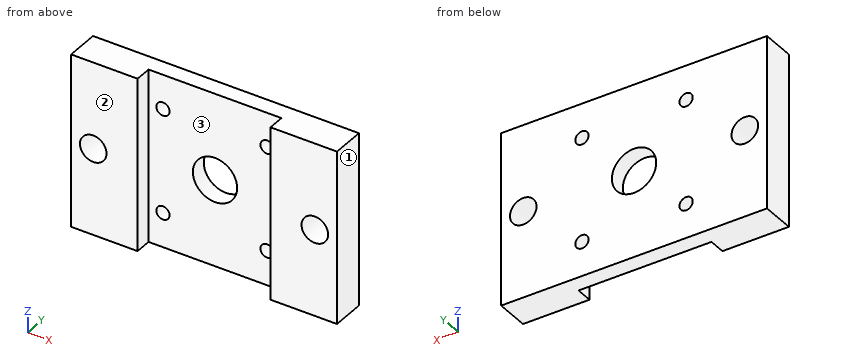
```python
from build123d import *

# Parameters (mm, degrees)
F0_W     = 120
F0_H     = 78
F0_R     = 6
F1_DEPTH = 15
F2_W     = 60
F2_H     = 78
F3_DEPTH = 7.5
F5_D     = 6
F7_D     = 20


with BuildPart() as f1:
    # F0 (on Front) → F1 (new body)
    with BuildSketch(Plane.XZ):
        with Locations((60, 39)):
            Rectangle(F0_W, F0_H)
        with Locations((10, 39)):
            Circle(F0_R, mode=Mode.SUBTRACT)
        with Locations((110, 39)):
            Circle(F0_R, mode=Mode.SUBTRACT)
    extrude(amount=F1_DEPTH)

    # F2 (on face) → F3 (cut)
    with BuildSketch(Plane.XZ.offset(15)):
        with Locations((60, 39)):
            Rectangle(F2_W, F2_H)
    extrude(amount=-F3_DEPTH, mode=Mode.SUBTRACT)

    # F5 (through all)
    with Locations(Plane.XZ.offset(7.5)):
        with Locations((36.5, 62.5), (36.5, 15.5), (83.5, 15.5), (83.5, 62.5)):
            Hole(F5_D / 2)

    # F7 (through all)
    with Locations(Plane.XZ.offset(7.5)):
        with Locations((60, 39)):
            Hole(F7_D / 2)


solid = f1.part
```
Could you check a few things on this model? Use its own coordinates, in mm. Face numbers are marked on the shaded views. Coordinates: 2 decimals unless noted, no trailing zeros. Write each loop counter-clockwise with the first axis right and the second up, starting at its lowest first coordinate (ties: lowest second). Pieces come first, ordered by that corner, then holes. Notation, with made-up numbers: (9.5, 5) - (31.5, 5) arc R21 cw to (31.5, 11) - close; hole circle Ø3 at (76, 87). An arc over 180 degrees is marked (long way). Use a Markdown table: item, result.
Q1. Imagine slicing it at C-C (x = 52). List the corners of the cut face in (y, z) for me, and give its area (3 significant figures).
Geometry check:
| item | result |
|---|---|
| outline | (-7.5, 0) - (0, 0) - (0, 33) - (-7.5, 33) - close; (-7.5, 45) - (0, 45) - (0, 78) - (-7.5, 78) - close |
| area | 495 mm2 |
Q2. I'm going to push flat-ended pins straight in: pin 1 Ø9.5 at (x, z) = (10, 39) entering from -Y; pin 2 Ø7 at (x, z) = (36.5, 15.5) entering from -Y. Where does each tip first touch, or does it pass through?
Geometry check:
| item | result |
|---|---|
| pin 1 | passes through |
| pin 2 | stops at y = -7.5 |
Q3. Please list where these lines run through material, in increasing order: L1, parallel to Z at x = 36.5, y = -4.5; L2, parallel to X at y = -12.5, z = 41; L3, parallel to X at y = -10.75, z = 30.
Geometry check:
| item | result |
|---|---|
| L1 | z = 0 to 12.5, 18.5 to 59.5, 65.5 to 78 |
| L2 | x = 0 to 4.34, 15.66 to 30, 90 to 104.34, 115.66 to 120 |
| L3 | x = 0 to 30, 90 to 120 |
Q4. Thinking about a two-plate mould opening in X: for the marked faces 1, 2 and 3, which applies, +X half, -X half, draft (parallel to the pull), parting line (faces both ways), or undercut?
Geometry check:
| item | result |
|---|---|
| face 1 | +X half |
| face 2 | draft |
| face 3 | undercut |
Q5. Imagine slicing it at B-B (z = 62.5). List the corners of the cut face in (x, y) for me.
Geometry check:
| item | result |
|---|---|
| outline | (0, -15) - (30, -15) - (30, -7.5) - (33.5, -7.5) - (33.5, 0) - (0, 0) - close; (39.5, -7.5) - (80.5, -7.5) - (80.5, 0) - (39.5, 0) - close; (86.5, -7.5) - (90, -7.5) - (90, -15) - (120, -15) - (120, 0) - (86.5, 0) - close |
Q6. Imagine slicing it at A-A (y = -11). List the corners of the cut face in (x, z) for me, and give its area (3 significant figures).
Geometry check:
| item | result |
|---|---|
| outline | (0, 0) - (30, 0) - (30, 78) - (0, 78) - close; (90, 0) - (120, 0) - (120, 78) - (90, 78) - close; hole circle Ø12 at (10, 39); hole circle Ø12 at (110, 39) |
| area | 4,450 mm2 |
Q7. Imagine slicing it at D-D (x = 36.5). List the corners of the cut face in (y, z) for me.
Geometry check:
| item | result |
|---|---|
| outline | (-7.5, 0) - (0, 0) - (0, 12.5) - (-7.5, 12.5) - close; (-7.5, 18.5) - (0, 18.5) - (0, 59.5) - (-7.5, 59.5) - close; (-7.5, 65.5) - (0, 65.5) - (0, 78) - (-7.5, 78) - close |
